Model file for the job. Use its own axes, mm. A direction names the side the tool comes from. Coordinates: 2 decimals unless noted, no trailing zeros. Write each loop counter-clockwise with the first axis right and the second up, starting at its lowest first coordinate (ties: lowest second). Pieces come first, ordered by that corner, then holes. Notation, with made-up numbers: M 6.25,-2.75 L 11.25,-2.75 A16 ccw 11.25,5.25 Z; hole C -5.5,-20 d4. An arc over 180 degrees is marked long. Put each result on its own line as item: value. Start each with the question number.
Q1. Drop flat-ended pins along their axis: pin 1 (4 mm diameter, centred on y = 34.5, z = -49, fed in from +X); pin 2 (4 mm diameter, centred on x = -4.5, z = 88, fed in from +Y); pin 3 (3.5 mm diameter, centred on x = -2, z = -21, fed in from -Y). Give the stop position or say it passes through.
Q2. Drill centre lines: line 1 along Y through (x, z) = (0, 81); line 2 along Z through (x, y) = (-43.5, -57.5); line 3 along Z through (x, y) = (56.5, 40). Where is each one in solid material? Low to high.
Q3. Which spindle directions (+Z, -Z, +X, -X, +Y, -Y) get a long thin tool onto all of the face, cutting with end or side? Do faces 1 (the flat face through (-9.149, -54, 87)), 2 (the flat face through (0, 27, 1)), 3 (the flat face through (-2, 68.901, 87)), 4 (the conical face through (-48.95, 37.53, 38.93)). Say none if no direction does.
Q4. Cut at A-A (z = 2). Write the cut outline in (x, y).
Q5. Pull direction Y, two halves, no side cores. Call faces 5 (the flat face through (-2, -38.901, 87)), 6 (the flat face through (-2, 38.901, 87)), 7 (the flat face through (-2, -68.901, 87)), 8 (the conical face through (58.832, -18.527, -25.072)): pulls with the +Y half, pulls with the -Y half, needs draft (parallel to the pull), parting line crosses it, or undercut.
```python
from build123d import *

# Parameters (mm, degrees)
SKETCH1_R           = 75
SKETCH1_R_2         = 24
BOSS_EXTRUDE1_DEPTH = 85
SKETCH3_W           = 12
SKETCH3_H           = 6
CUT_EXTRUDE1_DEPTH  = 201.374649095
SKETCH4_R           = 35
SKETCH4_R_2         = 20
CUT_EXTRUDE2_DEPTH  = 10
SKETCH5_W           = 15
SKETCH5_H           = 30
BOSS_EXTRUDE2_DEPTH = 5


with BuildPart() as part:
    # Sketch1 → Boss-Extrude1 (new, symmetric)
    with BuildSketch(Plane.XY):
        Circle(SKETCH1_R)
        Circle(SKETCH1_R_2, mode=Mode.SUBTRACT)
    extrude(amount=BOSS_EXTRUDE1_DEPTH, both=True)

    # Sketch2 → Cut-Revolve1 (revolve, cut)
    with BuildSketch(Plane(origin=(0, 0, 0), x_dir=(1, 0, 0), z_dir=(0, 1, 0))):
        Polygon((75, 75), (61, 70.71977046), (61, 57.28022954), (75, 53), align=None)
        Polygon((75, 43), (75, 21), (61, 25.28022954), (61, 38.71977046), align=None)
        Polygon((75, -21), (75, -43), (61, -38.71977046), (61, -25.28022954), align=None)
        Polygon((75, 11), (61, 6.71977046), (61, -6.71977046), (75, -11), align=None)
        Polygon((75, -75), (75, -53), (61, -57.28022954), (61, -70.71977046), align=None)
    revolve(axis=Axis((0, 0, 0), (0, 0, -1)), mode=Mode.SUBTRACT)

    # Sketch3 → Cut-Extrude1 (cut, through all)
    with BuildSketch(Plane.XY.offset(85)):
        with Locations((0, 24)):
            Rectangle(SKETCH3_W, SKETCH3_H)
    extrude(amount=-CUT_EXTRUDE1_DEPTH, mode=Mode.SUBTRACT)

    # Sketch4 → Cut-Extrude2 (cut)
    with BuildSketch(Plane.XY.offset(85)):
        Circle(SKETCH4_R)
        Circle(SKETCH4_R_2, mode=Mode.SUBTRACT)
    cut_extrude2 = extrude(amount=-CUT_EXTRUDE2_DEPTH, mode=Mode.SUBTRACT)

    # Mirror1: Cut-Extrude2 across plane
    add(cut_extrude2.mirror(Plane.XY), mode=Mode.SUBTRACT)

    # Sketch5 → Boss-Extrude2 (add)
    with BuildSketch(Plane.XY.offset(85)):
        with Locations((-1.649481041, 53.900577931)):
            Rectangle(SKETCH5_W, SKETCH5_H)
        with Locations((-1.649481041, -53.900577931)):
            Rectangle(SKETCH5_W, SKETCH5_H)
    extrude(amount=BOSS_EXTRUDE2_DEPTH)


solid = part.part
```
Computed values:
1. pin 1: x = 67.59
1. pin 2: y = 68.9
1. pin 3: y = -75
2. line 1: -75 to -35, 35 to 75
2. line 2: -85 to -74.11, -53.89 to -42.11, -21.89 to -10.11, 10.11 to 21.89, 42.11 to 53.89, 74.11 to 85
2. line 3: -85 to -73.23, -54.77 to -41.23, -22.77 to -9.23, 9.23 to 22.77, 41.23 to 54.77, 73.23 to 85
3. face 1: +Z, -X, +Y, -Y
3. face 2: +Z, -Z
3. face 3: +Z, +X, -X, +Y
3. face 4: none
4. outline: C 0,0 d122; hole M -6,23.24 A24 ccw long 6,23.24 L 6,27 L -6,27 Z
5. face 5: undercut
5. face 6: undercut
5. face 7: pulls with the -Y half
5. face 8: parting line crosses it
